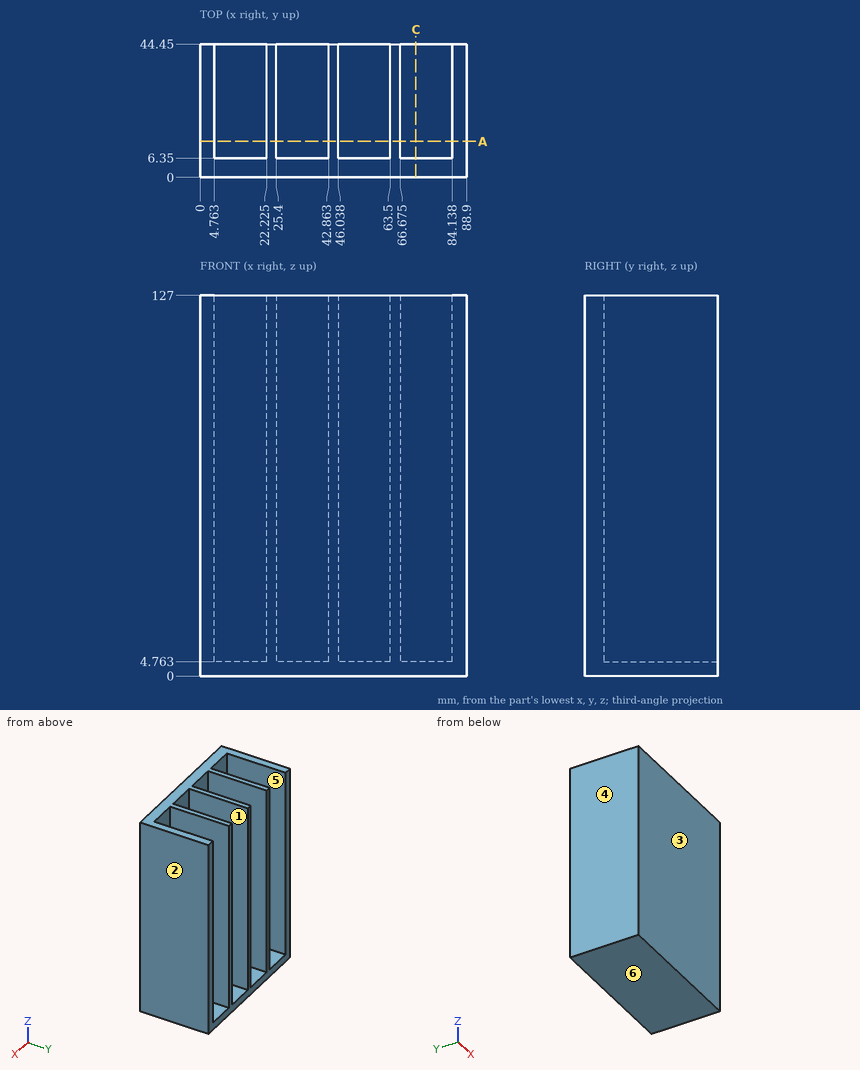
Print and shaded views of the part. All mm, measured from the part's lowest x, y and z. A direction names the side the tool comes from. Give positions to 0.01 mm unless a question says otherwise; leave off trailing zeros. Order: outer loops, then holes, each group sorted by start corner. A loop starts at its lowest first (then second) coordinate and runs counter-clockwise, first axis right, second up. Notation, with made-up numbers: (37, 76) - (75, 76) arc R7 ccw to (75, 86) - close; hole circle Ø6 at (61.5, -15). An arc over 180 degrees is marked (long way). Use a Markdown table: item, result.
1) Two-plate mould, pull along X, no slides. Class the marked faces 1, 2, 3 and 4: +X half, -X half, draft (parallel to the pull), parting line (faces both ways), or undercut.
Checked values:
| item | result |
|---|---|
| face 1 | undercut |
| face 2 | +X half |
| face 3 | draft |
| face 4 | -X half |
2) Probe L1, parallel to X at y = 27, z = 28.5 (1 decimal); L2, parallel to Y at x = 30, z = 48; L3, parallel to Z at x = 53.5, y = 19. List the from-to ranges inside material, lowest first. Write a range as from..to.
Checked values:
| item | result |
|---|---|
| L1 | 0..4.8, 22.2..25.4, 42.9..46, 63.5..66.7, 84.1..88.9 |
| L2 | 0..6.35 |
| L3 | 0..4.76 |
3) Flat gauge pins, fed straight in: P1, Ø8.5, axis at x = 37.5, y = 33, coming from the +Z side; P2, Ø5, axis at x = 71.5, z = 82.5, coming from the +Y side. Where does each tip first touch, or does it go through?
Checked values:
| item | result |
|---|---|
| P1 | z = 4.76 |
| P2 | y = 6.35 |
4) Saw through at A-A on y = 12. List the corners of the cut face in (x, z) (1 decimal), plus the area to 3 significant figures.
Checked values:
| item | result |
|---|---|
| outline | (0, 0) - (88.9, 0) - (88.9, 127) - (84.1, 127) - (84.1, 4.8) - (66.7, 4.8) - (66.7, 127) - (63.5, 127) - (63.5, 4.8) - (46, 4.8) - (46, 127) - (42.9, 127) - (42.9, 4.8) - (25.4, 4.8) - (25.4, 127) - (22.2, 127) - (22.2, 4.8) - (4.8, 4.8) - (4.8, 127) - (0, 127) - close |
| area | 2,750 mm² |
5) 3-axis set-ups, long thin cutter, end or side, ignore diameter. For the marked faces 5 and 6: which of +Z, -Z, +X, -X, +Y, -Y reach the whole face in a straight line?
Checked values:
| item | result |
|---|---|
| face 5 | +Z, +Y |
| face 6 | -Z, +X, -X, +Y, -Y |
6) Saw through at C-C on x = 72. List the corners of the cut face in (y, z).
Checked values:
| item | result |
|---|---|
| outline | (0, 0) - (44.45, 0) - (44.45, 4.76) - (6.35, 4.76) - (6.35, 127) - (0, 127) - close |
